The listing builds one solid part. Answer for the finished solid, in the listing's coordinates (mm). Face numbers are marked on the shaded views. Give positions to 0.01 mm unless a question says otherwise; leave off trailing zeros. Loops run counter-clockwise (first coordinate to the right, second up) from the corner with the lowest first, then second, coordinate; pieces in that order, holes last. Notation, with made-up numbers: M -33,-12.75 L 1,-12.75 A29 ccw 1,21.25 Z; hole C 48.5,49 d10. An arc over 180 degrees is marked long. Return JSON: item names as keys, results as strings.
from build123d import *

# Parameters (mm, degrees)
CIRCLE_R                     = 2
BOSS_EXTRU_1_DEPTH           = 40.2
ENL_V_MAT_EXTRU_1_DEPTH      = 4
ENL_V_MAT_EXTRU_2_DEPTH      = 5
GORGECIRCLIPPOLULU_OUTSIDE_W = 14.12
GORGECIRCLIPPOLULU_OUTSIDE_H = 14.12
GORGECIRCLIPPOLULU_OUTSIDE_R = 1.9
ENL_V_MAT_EXTRU_3_DEPTH      = 0.5
ESQUISSE1_OUTSIDE_W          = 14.12
ESQUISSE1_OUTSIDE_H          = 14.12
ESQUISSE1_OUTSIDE_R          = 1.9
ENL_V_MAT_EXTRU_4_DEPTH      = 0.5
CHANFREIN1_SIZE              = 0.25
CHANFREIN2_SIZE              = 0.25


with BuildPart() as part:
    # Circle → Boss.-Extru.1 (new body)
    with BuildSketch(Plane.XY):
        Circle(CIRCLE_R)
    extrude(amount=BOSS_EXTRU_1_DEPTH)

    # MeplatPololu → Enlèv. mat.-Extru.1 (cut)
    with BuildSketch(Plane.XY.offset(37.6)):
        with BuildLine():
            Line((-1.6, 1.2), (1.6, 1.2))
            ThreePointArc((1.6, 1.2), (0, 2), (-1.6, 1.2))
        make_face()
    extrude(amount=-ENL_V_MAT_EXTRU_1_DEPTH, mode=Mode.SUBTRACT)

    # MeplatRoueDentee → Enlèv. mat.-Extru.2 (cut)
    with BuildSketch(Plane.XY.offset(17.09)):
        with BuildLine():
            Line((0.164576352, -1.993217154), (-1.959569847, 0.400107505))
            ThreePointArc((-1.959569847, 0.400107505), (-1.495827912, -1.327591374), (0.164576352, -1.993217154))
        make_face()
    extrude(amount=-ENL_V_MAT_EXTRU_2_DEPTH, mode=Mode.SUBTRACT)

    # GorgeCirclipPolulu outside → Enlèv. mat.-Extru.3 (cut)
    with BuildSketch(Plane.XY.offset(38.7)):
        Rectangle(GORGECIRCLIPPOLULU_OUTSIDE_W, GORGECIRCLIPPOLULU_OUTSIDE_H)
        Circle(GORGECIRCLIPPOLULU_OUTSIDE_R, mode=Mode.SUBTRACT)
    extrude(amount=ENL_V_MAT_EXTRU_3_DEPTH, mode=Mode.SUBTRACT)

    # Esquisse1 outside → Enlèv. mat.-Extru.4 (cut)
    with BuildSketch(Plane.XY.offset(8.99)):
        Rectangle(ESQUISSE1_OUTSIDE_W, ESQUISSE1_OUTSIDE_H)
        Circle(ESQUISSE1_OUTSIDE_R, mode=Mode.SUBTRACT)
    extrude(amount=-ENL_V_MAT_EXTRU_4_DEPTH, mode=Mode.SUBTRACT)

    # Chanfrein1
    chanfrein1_edges = [part.edges().sort_by_distance(p)[0] for p in [
        (-2, 0, 40.2),
    ]]
    chamfer(chanfrein1_edges, length=CHANFREIN1_SIZE)

    # Chanfrein2
    chanfrein2_edges = [part.edges().sort_by_distance(p)[0] for p in [
        (-2, 0, 0),
    ]]
    chamfer(chanfrein2_edges, length=CHANFREIN2_SIZE)


solid = part.part
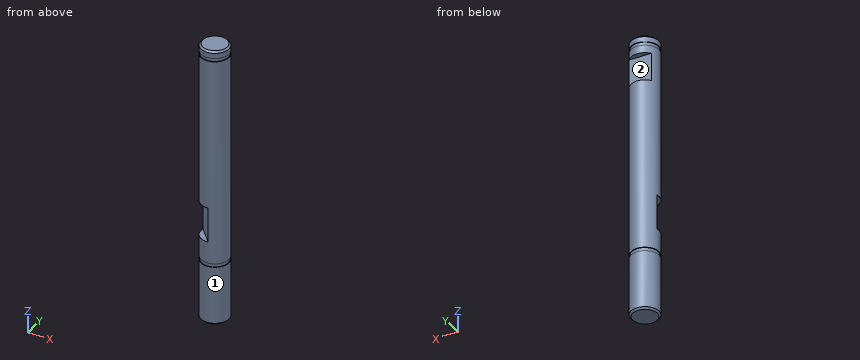
(1) Determine the mould class of the marked faces 1 and 2 for opening direction Z: released by +Z, released by -Z, zero draft, split by the parting line, or undercut.
Values follow:
{"face 1": "zero draft", "face 2": "undercut"}
(2) The part is cut by section A-A (z = 29.5). Determine the outline of the cut face in (x, y).
Values follow:
{"outline": "C 0,0 d4"}
(3) Straight lines are drawn through the part: line 1 along Z through (x, y) = (-0.9, 1.4); line 2 along Z through (x, y) = (0.95, -1.7); line 3 along X through (y, z) = (0.1, 27). For each, find the intervals that lie inside material, in ascending order.
Values follow:
{"line 1": "0 to 33.6, 37.6 to 40.2", "line 2": "0.2 to 8.49, 8.99 to 38.7, 39.2 to 40", "line 3": "-2 to 2"}
(4) The part is cut by section B-B (z = 14.5). Determine the outline of the cut face in (x, y), and give its area (3 significant figures).
Values follow:
{"outline": "M -1.96,0.4 L 0.16,-1.99 A2 ccw long Z", "area": "10.8 mm²"}
(5) Given pin 1 (2 mm diameter, centred on x = 0, y = 0.5, fed in from -Z); pin 2 (1 mm diameter, centred on y = -1, z = 28, fed in from -X), each flat-ended and moving along its own axis, determine where each tip first touches the part or whether it passes through.
Values follow:
{"pin 1": "z = 0", "pin 2": "x = -1.94"}
